```python
from build123d import *

# Parameters (mm, degrees)
SKETCH_1_R      = 1.25
EXTRUDE_1_DEPTH = 20


with BuildPart() as part:
    # Эскиз1 → Бобышка-Вытянуть1 (new body)
    with BuildSketch(Plane(origin=(0, 0, 0), x_dir=(1, 0, 0), z_dir=(0, 1, 0))):
        with BuildLine():
            Line((-2, -2.5), (2, -2.5))
            ThreePointArc((2, -2.5), (2.353553391, -2.353553391), (2.5, -2))
            Line((2.5, -2), (2.5, 2))
            ThreePointArc((2.5, 2), (2.353553391, 2.353553391), (2, 2.5))
            Line((2, 2.5), (-2, 2.5))
            ThreePointArc((-2, 2.5), (-2.353553391, 2.353553391), (-2.5, 2))
            Line((-2.5, 2), (-2.5, -2))
            ThreePointArc((-2.5, -2), (-2.353553391, -2.353553391), (-2, -2.5))
        make_face()
        with Locations(Location((0, 0, 0), (0, 0, 270))):
            Circle(SKETCH_1_R, mode=Mode.SUBTRACT)
    extrude(amount=EXTRUDE_1_DEPTH)

    # Бобышка-Вытянуть2 cone 1 section (through the dimple's axis) → Бобышка-Вытянуть2 (revolve)
    with BuildSketch(Plane(origin=(0, 0, 0), x_dir=(0, 0, 1), z_dir=(1, 0, 0))):
        Polygon((0, 0), (4, 0), (0, 1.950930354), align=None)
    revolve(axis=Axis((0, 0, 0), (0, -1, 0)))


solid = part.part
```
The listing builds one solid part. Answer for the finished solid, in the listing's coordinates (mm). A direction names the side the tool comes from. Coordinates: 2 decimals unless noted, no trailing zeros. Loops run counter-clockwise (first coordinate to the right, second up) from the corner with the lowest first, then second, coordinate; pieces in that order, holes last. Notation, with made-up numbers: (-0.5, 37) - (7.5, 37) arc R15 cw to (7.5, 62) - close; hole circle Ø5 at (-27.5, 12). An arc over 180 degrees is marked (long way). Use a Markdown table: item, result. Add a question column.
1) The part is cut by section A-A, the plane y = 16. Give the vertices of the cut face in (x, z).
2) For faces 4 (the flat face through (0, 0, -3)), 5 (the flat face through (2.5, 10, 0)), 6 (the flat face through (-2.5, 10, 0)), determine the directions among +Z, -Z, +X, -X, +Y, -Y from which every point of the face is accessible in a straight line to the end or side of a thin tool.
3) Given pin 1 (2 mm diameter, centred on x = 0.5, y = 6.5, fed in from -Z); pin 2 (4.5 mm diameter, centred on y = 12.5, z = 1, fed in from +X); pin 3 (3 mm diameter, centred on x = 0, z = 0, fed in from +Y); pin 4 (2 mm diameter, centred on y = 13.5, z = 0, fed in from -X), each flat-ended and moving along its own axis, determine where each tip first touches the part or whether it passes through.
4) Find the intervals of material crossed by line 1 (X direction, y = 12.75, z = 0); line 2 (X direction, y = 0.5, z = 0.75); line 3 (Z direction, x = 0.25, y = 18.5), in increasing order.
5) The mould has two halves that part along X. Classify faces 1 (the flat face through (0, 10, -2.5)), 2 (the flat face through (0, 0, 0)), 3 (the conical face through (-0.058, -1.856, 0.185)): released by +X, released by -X, zero draft, split by the parting line, or undercut.
Here are the results:
| question | item | result |
|---|---|---|
| 1 | outline | (-2.5, -2) arc R0.5 ccw to (-2, -2.5) - (2, -2.5) arc R0.5 ccw to (2.5, -2) - (2.5, 2) arc R0.5 ccw to (2, 2.5) - (-2, 2.5) arc R0.5 ccw to (-2.5, 2) - close; hole circle Ø2.5 at (0, 0) |
| 2 | face 4 | +Y |
| 2 | face 5 | +Z, -Z, +X, +Y |
| 2 | face 6 | +Z, -Z, -X, +Y |
| 3 | pin 1 | stops at z = -2.5 |
| 3 | pin 2 | stops at x = 2.5 |
| 3 | pin 3 | stops at y = 20 |
| 3 | pin 4 | stops at x = -2.5 |
| 4 | line 1 | x = -2.5 to -1.25, 1.25 to 2.5 |
| 4 | line 2 | x = -2.5 to -1, 1 to 2.5 |
| 4 | line 3 | z = -2.5 to -1.22, 1.22 to 2.5 |
| 5 | face 1 | zero draft |
| 5 | face 2 | undercut |
| 5 | face 3 | split by the parting line |
